Could you check a few things on this model? Use its own coordinates, in mm. A direction names the side the tool comes from. Coordinates: 2 decimals unless noted, no trailing zeros. Write each loop counter-clockwise with the first axis right and the second up, starting at its lowest first coordinate (ties: lowest second). Pieces come first, ordered by that corner, then holes.
```python
from build123d import *

# Parameters (mm, degrees)
F0_W           = 75
F0_H           = 75
F0_R           = 18.625
F1_DEPTH       = 3
F2_DEPTH       = 75
F3_R           = 18.625
F4_DEPTH       = 10.2
F0_W_2         = 15
F0_H_2         = 2.5
F5_DEPTH       = 77
F6_W           = 72
F6_H           = 72
F7_DEPTH       = 4
F8_SIZE        = 1
F10_W          = 12.5
F10_H          = 25
F11_DEPTH      = 25
F9_W           = 15
F9_H           = 25
F12_DEPTH      = 14.8
F14_DEPTH      = 3.8
F15_R          = 1.5
F15_R_2        = 4.25
F15_W          = 11.1
F15_H          = 5.7
F15_R_3        = 3
F16_DEPTH      = 25
F16_DEPTH_BACK = 25
F17_SIZE2      = 2
F17_SIZE       = 2


# Not quite as in the source:
# - a feature names something its author has since deleted; it is built from what else it names


with BuildPart() as f1:
    # F0 (on Top) → F1 (new body)
    with BuildSketch(Plane.XY):
        Rectangle(F0_W, F0_H)
        Polygon((-34.5, 12.5), (-34.5, 34.5), (29, 34.5), (31.5, 34.5), (34.5, 34.5), (34.5, -34.5), (-34.5, -34.5), (-34.5, 10), align=None, mode=Mode.SUBTRACT)
        Polygon((29, 34.5), (-34.5, 34.5), (-34.5, 12.5), (-19.5, 12.5), (-19.5, 10), (-34.5, 10), (-34.5, -34.5), (34.5, -34.5), (34.5, 34.5), (31.5, 34.5), (31.5, 10), (16.5, 10), (16.5, 12.5), (29, 12.5), align=None)
        Circle(F0_R, mode=Mode.SUBTRACT)
    extrude(amount=F1_DEPTH)

    # F0 (on Top) → F2 (join)
    with BuildSketch(Plane.XY):
        Rectangle(F0_W, F0_H)
        Polygon((-34.5, 12.5), (-34.5, 34.5), (29, 34.5), (31.5, 34.5), (34.5, 34.5), (34.5, -34.5), (-34.5, -34.5), (-34.5, 10), align=None, mode=Mode.SUBTRACT)
    extrude(amount=F2_DEPTH)

    # F3 (on face) → F4 (cut)
    with BuildSketch(Plane.XZ.offset(37.5)):
        with Locations((0, 37.5)):
            Circle(F3_R)
    extrude(amount=-F4_DEPTH, mode=Mode.SUBTRACT)

    # F0 (on Top) → F5 (join)
    with BuildSketch(Plane.XY):
        with Locations((-27, 11.25)):
            Rectangle(F0_W_2, F0_H_2)
        Polygon((31.5, 34.5), (29, 34.5), (29, 12.5), (16.5, 12.5), (16.5, 10), (31.5, 10), align=None)
    extrude(amount=F5_DEPTH)

    # F6 (on face) → F7 (cut)
    with BuildSketch(Plane.XY.offset(75)):
        Rectangle(F6_W, F6_H)
        Polygon((-34.5, 10), (-34.5, 12.5), (-34.5, 34.5), (29, 34.5), (31.5, 34.5), (34.5, 34.5), (34.5, -34.5), (-34.5, -34.5), align=None, mode=Mode.SUBTRACT)
    extrude(amount=-F7_DEPTH, mode=Mode.SUBTRACT)

    # F8
    f8_edges = [f1.edges().sort_by_distance(p)[0] for p in [
        (37.5, 0, 0),
        (0, -37.5, 0),
        (-37.5, -37.5, 37.5),
        (37.5, -37.5, 37.5),
        (-37.5, 0, 0),
        (0, 37.5, 0),
        (37.5, 37.5, 37.5),
        (-37.5, 37.5, 37.5),
    ]]
    chamfer(f8_edges, length=F8_SIZE)

    # F10 (on face) → F11 (cut)
    with BuildSketch(Plane(origin=(0, 12.5, 0), x_dir=(-1, 0, 0), z_dir=(0, 1, 0))):
        with Locations((-22.75, 64.5)):
            Rectangle(F10_W, F10_H)
        with Locations((-22.75, 15.5)):
            Rectangle(F10_W, F10_H)
    extrude(amount=-F11_DEPTH, mode=Mode.SUBTRACT)

    # F9 (on face) → F12 (cut)
    with BuildSketch(Plane.XZ.offset(-10)):
        Polygon((-19.5, 77), (-34.5, 77), (-34.5, 71), (-34.5, 52), (-19.5, 52), align=None)
        with Locations((-27, 15.5)):
            Rectangle(F9_W, F9_H)
    extrude(amount=-F12_DEPTH, mode=Mode.SUBTRACT)

    # F13 (on face) → F14 (cut)
    with BuildSketch(Plane(origin=(29, 0, 0), x_dir=(0, -1, 0), z_dir=(-1, 0, 0))):
        Polygon((-12.5, 52), (-10, 52), (-10, 77), (-34.5, 77), (-34.5, 71), (-34.5, 52), align=None)
        Polygon((-10, 28), (-12.5, 28), (-34.5, 28), (-34.5, 3), (-10, 3), align=None)
    extrude(amount=-F14_DEPTH, mode=Mode.SUBTRACT)

    # F15 (on face) → F16 (cut, two sides)
    with BuildSketch(Plane.YZ.offset(37.5)) as f16_sk:
        with Locations((-30.8012962341, 20)):
            Circle(F15_R)
        with Locations((-17.5, 20)):
            Circle(F15_R_2)
        with Locations((-17.5, 10)):
            Rectangle(F15_W, F15_H)
        with Locations((-30.8012962341, 10)):
            Circle(F15_R_3)
    extrude(amount=-F16_DEPTH, mode=Mode.SUBTRACT)
    extrude(f16_sk.sketch, amount=F16_DEPTH_BACK, mode=Mode.SUBTRACT)

    # F17
    f17_edges = [f1.edges().sort_by_distance(p)[0] for p in [
        (16.5, 10, 40),
        (24, 10, 52),
        (-27, 10, 52),
        (-19.5, 10, 40),
        (31.5, 22.25, 52),
    ]]
    chamfer(f17_edges, length=F17_SIZE, length2=F17_SIZE2)


solid = f1.part
```
1. I want a section at C-C on y = -17.5. Please give me the cut outline in (x, z) (3 decimals), plus the area to 3 significant figures.
Verdict:
outline: (-37.5, 1) - (-36.5, 0) - (-6.375, 0) - (-6.375, 3) - (-34.5, 3) - (-34.5, 71) - (-36, 71) - (-36, 75) - (-37.5, 75) - close; (6.375, 0) - (36.5, 0) - (37.5, 1) - (37.5, 7.15) - (34.5, 7.15) - (34.5, 3) - (6.375, 3) - close; (34.5, 12.85) - (37.5, 12.85) - (37.5, 15.75) - (34.5, 15.75) - close; (34.5, 24.25) - (37.5, 24.25) - (37.5, 75) - (36, 75) - (36, 71) - (34.5, 71) - close
area: 563 mm2
2. I want a section at D-D on x = -26. Please give me the cut outline in (y, z), plus the area to 3 significant figures.
Verdict:
outline: (-37.5, 1) - (-36.5, 0) - (36.5, 0) - (37.5, 1) - (37.5, 75) - (36, 75) - (36, 71) - (34.5, 71) - (34.5, 3) - (-34.5, 3) - (-34.5, 71) - (-36, 71) - (-36, 75) - (-37.5, 75) - close; (10, 28) - (12.5, 28) - (12.5, 52) - (12, 52) - (10, 50) - close
area: 702 mm2
3. For pin 1 (3 mm diameter, centred on x = 6, z = 55, fed in from -Y); pin 2 (3 mm diameter, centred on x = -28, y = 25, fed in from +Z); pin 3 (10.5 mm diameter, centred on x = 21, y = 17.5, fed in from +Z), each with a flat end and sliding along its axis, tell me the tip position at first contact or that it passes through.
Verdict:
pin 1: stops at y = -37.5
pin 2: stops at z = 3
pin 3: stops at z = 52
4. On a 3-axis mill with a long thin cutter (end or side, diameter ignored), from which of +Z, -Z, +X, -X, +Y, -Y can I reach the whole of each face in a straight line? I mean faces 4 (the face through (-27, 11, 28)), 5 (the face through (-27, 11, 51)), 6 (the face through (36.02, -18.42, 15.85)). Say none if no direction works.
Verdict:
face 4: none
face 5: +Z
face 6: +X
5. Please list where these lines run through material, in increasing order: line 1 along Y through (x, z) = (20, 35.5); line 2 along X through (y, z) = (3, 39.5).
Verdict:
line 1: y = -37.5 to -34.5, 10 to 12.5, 34.5 to 37.5
line 2: x = -37.5 to -34.5, 34.5 to 37.5
6. I want a section at B-B on x = 0. Please give me the cut outline in (y, z) (3 decimals), plus the area to 4 significant figures.
Verdict:
outline: (-37.5, 1) - (-36.5, 0) - (-18.625, 0) - (-18.625, 3) - (-34.5, 3) - (-34.5, 18.875) - (-37.5, 18.875) - close; (-37.5, 56.125) - (-34.5, 56.125) - (-34.5, 71) - (-36, 71) - (-36, 75) - (-37.5, 75) - close; (18.625, 0) - (36.5, 0) - (37.5, 1) - (37.5, 75) - (36, 75) - (36, 71) - (34.5, 71) - (34.5, 3) - (18.625, 3) - close
area: 420.5 mm2
7. I want a section at A-A on z = 64.5. Please give me the cut outline in (x, y), plus the area to 3 significant figures.
Verdict:
outline: (-37.5, -36.5) - (-36.5, -37.5) - (36.5, -37.5) - (37.5, -36.5) - (37.5, 36.5) - (36.5, 37.5) - (-36.5, 37.5) - (-37.5, 36.5) - close; hole (-34.5, -34.5) - (34.5, -34.5) - (34.5, 34.5) - (-34.5, 34.5) - close
area: 862 mm2
8. If we mould it in two halves opening along Y, with no side actions, what happens to faces 1 (the face through (-1, 37.5, 37)), 2 (the face through (36, -18, 12.85)), 3 (the face through (-17, -37.5, 29))? For each: pulls with the +Y half, pulls with the -Y half, needs draft (parallel to the pull), parting line crosses it, or undercut.
Verdict:
face 1: pulls with the +Y half
face 2: undercut
face 3: pulls with the -Y half
